from build123d import *

# Parameters (mm, degrees)
EXTRUDE_1_DEPTH = 12.7


with BuildPart() as part:
    # 스케치1 → 보스-돌출1 (new body)
    with BuildSketch(Plane.XY):
        with BuildLine():
            ThreePointArc((-19.05, 36.398522628), (-34.380256121, 34.380256121), (-36.398522628, 19.05))
            ThreePointArc((-36.398522628, 19.05), (-31.294090512, 0), (-36.398522628, -19.05))
            ThreePointArc((-36.398522628, -19.05), (-34.380256121, -34.380256121), (-19.05, -36.398522628))
            ThreePointArc((-19.05, -36.398522628), (0, -31.294090512), (19.05, -36.398522628))
            ThreePointArc((19.05, -36.398522628), (34.380256121, -34.380256121), (36.398522628, -19.05))
            ThreePointArc((36.398522628, -19.05), (31.294090512, 0), (36.398522628, 19.05))
            ThreePointArc((36.398522628, 19.05), (34.380256121, 34.380256121), (19.05, 36.398522628))
            ThreePointArc((19.05, 36.398522628), (0, 31.294090512), (-19.05, 36.398522628))
        make_face()
    extrude(amount=-EXTRUDE_1_DEPTH)


solid = part.part
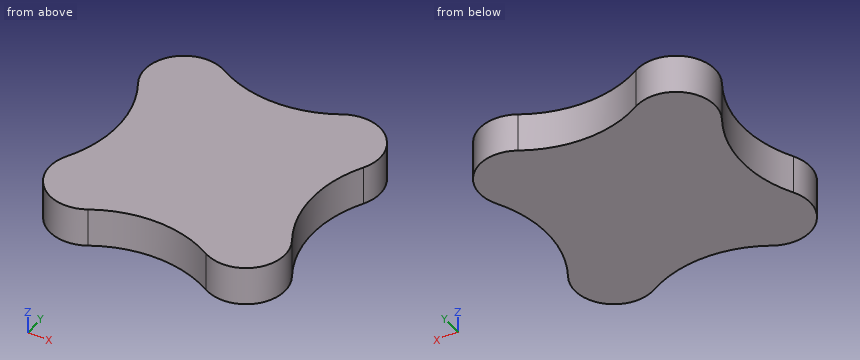
Model file for the job. Use its own axes, mm. Give positions to 0.01 mm unless a question says otherwise; leave off trailing zeros. Order: outer loops, then holes, each group sorted by start corner. A loop starts at its lowest first (then second) coordinate and runs counter-clockwise, first axis right, second up. Notation, with made-up numbers: M -15.75,25.25 L 12.25,25.25 A27 ccw 12.25,43.25 Z; hole C 29.25,45 d2. An arc over 180 degrees is marked long. Put each result on its own line as item: value. Start each with the question number.
(1) Drill centre lines: L1, parallel to Y at x = -0.5, z = -2; L2, parallel to X at y = 25, z = -9.75. Where is each one in solid material? Low to high. Write a range as [from, to].
(2) Pin check, flat tips, straight feed: pin 1 Ø5 at (y, z) = (-0.5, -7.5) entering from -X; pin 2 Ø2 at (y, z) = (-11, -3.5) entering from +X; pin 3 Ø6 at (x, z) = (21, -10.5) entering from +Y. Stop position of each tip, or through.
(3) Band-saw the part on C-C on x = -6.5. Give the cut face in (y, z).
(4) Band-saw the part on A-A on y = -33. Give the cut face in (x, z), then the cut area to 3 significant figures.
(5) Band-saw the part on D-D on y = -4. Give the cut face in (x, z).
(6) Band-saw the part on B-B on z = -1.25. Give the cut face in (x, y), then the cut area to 3 significant figures.
Results below:
1. L1: y = [-31.3, 31.3]
1. L2: x = [-38.09, 38.09]
2. pin 1: stops at x = -31.41
2. pin 2: stops at x = 33.23
2. pin 3: stops at y = 38.02
3. outline: M -31.85,-12.7 L 31.85,-12.7 L 31.85,0 L -31.85,0 Z
4. outline: M -35.57,-12.7 L -11.27,-12.7 L -11.27,0 L -35.57,0 Z; M 11.27,-12.7 L 35.57,-12.7 L 35.57,0 L 11.27,0 Z
4. area: 617 mm2
5. outline: M -31.5,-12.7 L 31.5,-12.7 L 31.5,0 L -31.5,0 Z
6. outline: M -36.4,-19.05 A12.7 ccw -19.05,-36.4 A38.1 cw 19.05,-36.4 A12.7 ccw 36.4,-19.05 A38.1 cw 36.4,19.05 A12.7 ccw 19.05,36.4 A38.1 cw -19.05,36.4 A12.7 ccw -36.4,19.05 A38.1 cw Z
6. area: 4,850 mm2
